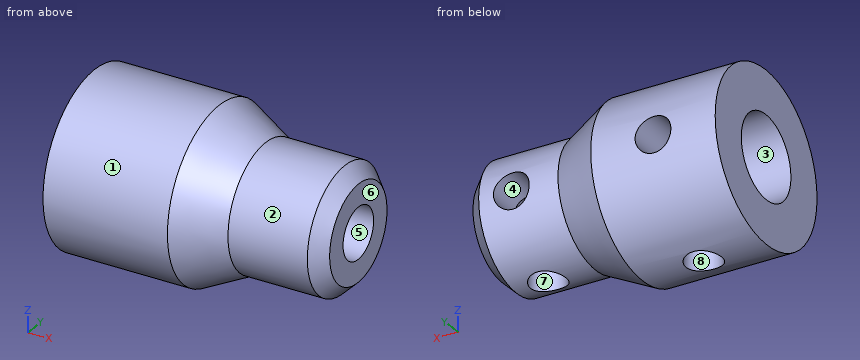
from build123d import *

# Parameters (mm, degrees)
SKETCH2_R          = 1.4605
CUT_EXTRUDE1_DEPTH = 16.107129112
CIRPATTERN1_COUNT  = 2
CIRPATTERN1_ANGLE  = 90
CHAMFER1_SIZE      = 1.143


with BuildPart() as part:
    # Sketch1 → Revolve1 (revolve)
    with BuildSketch(Plane(origin=(0, 0, 0), x_dir=(1, 0, 0), z_dir=(0, 1, 0)), mode=Mode.PRIVATE) as revolve1_sk:
        Polygon((-10.16, 3.4036), (0, 3.4036), (1.905, 2.0955), (11.43, 2.0955), (11.43, 5.08), (3.81, 5.08), (0, 6.985), (-10.16, 6.985), align=None)
    revolve(revolve1_sk.sketch.rotate(Axis((0, 0, 0), (1, 0, 0)), 180), axis=Axis((0, 0, 0), (1, 0, 0)))

    # Sketch2 → Cut-Extrude1 (cut, through all)
    with BuildSketch(Plane(origin=(0, 0, 0), x_dir=(1, 0, 0), z_dir=(0, 1, 0))):
        with Locations(Location((-5.08, 0, 0), (0, 0, 90))):
            Circle(SKETCH2_R)
        with Locations(Location((7.62, 0, 0), (0, 0, 90))):
            Circle(SKETCH2_R)
    cut_extrude1 = extrude(amount=CUT_EXTRUDE1_DEPTH, mode=Mode.SUBTRACT)

    # CirPattern1: Cut-Extrude1 ×2 about axis
    cirpattern1_axis = Axis((-10.16, 0, 0), (-1, 0, 0))
    for i in range(1, CIRPATTERN1_COUNT):
        add(cut_extrude1.rotate(cirpattern1_axis, i * CIRPATTERN1_ANGLE / (CIRPATTERN1_COUNT - 1)), mode=Mode.SUBTRACT)

    # Chamfer1
    chamfer1_edges = [part.edges().sort_by_distance(p)[0] for p in [
        (11.43, 0, -5.08),
    ]]
    chamfer(chamfer1_edges, length=CHAMFER1_SIZE)


solid = part.part
Geometry: final body of the model. Coordinates: model frame, mm. Face numbers are marked on the shaded views. A direction names the side the tool comes from. Give positions to 0.01 mm unless a question says otherwise; leave off trailing zeros. Write each loop counter-clockwise with the first axis right and the second up, starting at its lowest first coordinate (ties: lowest second). Pieces come first, ordered by that corner, then holes. Notation, with made-up numbers: M -17.75,-12 L 40.25,-12 A21 ccw 40.25,-5 Z; hole C 23.5,12 d10. An arc over 180 degrees is marked long. Answer in a Markdown table with one row per item. Add a question column.
(1) Section A-A on y = 0. Return loops of the section in (x, z) (1 decimal), and give its area (3 significant figures).
(2) Reachability of the marked faces 1, 2, 3 and 4 from +Z, -Z, +X, -X, +Y, -Y: full face, straight path, thin tool, end or side. Return the list, or none.
(3) First-contact query: pin 1 (3.5 mm diameter, centred on x = 7.62, z = 0, fed in from -Y); pin 2 (5.5 mm diameter, centred on y = 0, z = 0, fed in from -X); pin 3 (1 mm diameter, centred on x = 4, y = 0.5, fed in from +Z). Flat tips, straight axial feed; report the tip coordinate or a pass-through.
(4) Section B-B on z = 0. Return loops of the section in (x, y) (1 decimal), and give its area (3 significant figures).
(5) Section D-D on x = -3. Return loops of the section in (y, z) (3 decimals), and give its area (3 significant figures).
(6) Mould query, pull axis X, two halves, no side actions, for the marked faces 5, 6, 7 and 8. Classes: +X half, -X half, draft (parallel to the pull), parting line (faces both ways), or undercut.
(7) Ray query, line 1 (X direction, y = 0, z = -3.8); line 2 (X direction, y = 0, z = -3.35); line 3 (Z direction, x = -4, y = -2.5). Return the intervals inside material, ascending.
Result set:
| question | item | result |
|---|---|---|
| 1 | outline | M -10.2,-7 L -6.5,-7 L -6.5,-3.4 L -10.2,-3.4 Z; M -10.2,3.4 L 0,3.4 L 1.9,2.1 L 11.4,2.1 L 11.4,3.9 L 10.3,5.1 L 3.8,5.1 L 0,7 L -10.2,7 Z; M -3.6,-7 L 0,-7 L 3.8,-5.1 L 6.2,-5.1 L 6.2,-2.1 L 1.9,-2.1 L 0,-3.4 L -3.6,-3.4 Z; M 9.1,-5.1 L 10.3,-5.1 L 11.4,-3.9 L 11.4,-2.1 L 9.1,-2.1 Z |
| 1 | area | 125 mm^2 |
| 2 | face 1 | +X, -X |
| 2 | face 2 | +X |
| 2 | face 3 | -X |
| 2 | face 4 | +Y |
| 3 | pin 1 | stops at y = -5.08 |
| 3 | pin 2 | stops at x = 0.95 |
| 3 | pin 3 | stops at z = 5.21 |
| 4 | outline | M -10.2,-7 L 0,-7 L 3.8,-5.1 L 10.3,-5.1 L 11.4,-3.9 L 11.4,-2.1 L 1.9,-2.1 L 0,-3.4 L -10.2,-3.4 Z; M -10.2,3.4 L -6.5,3.4 L -6.5,7 L -10.2,7 Z; M -3.6,3.4 L 0,3.4 L 1.9,2.1 L 6.2,2.1 L 6.2,5.1 L 3.8,5.1 L 0,7 L -3.6,7 Z; M 9.1,2.1 L 11.4,2.1 L 11.4,3.9 L 10.3,5.1 L 9.1,5.1 Z |
| 4 | area | 125 mm^2 |
| 5 | outline | C 0,0 d13.97; hole C 0,0 d6.807 |
| 5 | area | 117 mm^2 |
| 6 | face 5 | draft |
| 6 | face 6 | +X half |
| 6 | face 7 | undercut |
| 6 | face 8 | undercut |
| 7 | line 1 | x = -10.16 to -6.54, -3.62 to 6.16, 9.08 to 11.43 |
| 7 | line 2 | x = 0.08 to 6.16, 9.08 to 11.43 |
| 7 | line 3 | z = -6.52 to -2.31, 2.31 to 6.52 |
